from build123d import *

# Parameters (mm, degrees)
F1_DEPTH    = 2.54
F2_R        = 1.905
F3_T2_ANGLE = 165.8998366825


# Not quite as in the source:
# - a fillet or chamfer that OpenCascade refuses, or shapes differently, is made with other operations: its cross-section is extruded or revolved along the edge and cut away or added


with BuildPart() as f1:
    # F0 (on Top) → F1 (new body)
    with BuildSketch(Plane.XY):
        with BuildLine():
            Line((0, -6.35), (0, 0))
            Line((0, 0), (-2.9618976002, 7.0207950124))
            ThreePointArc((-2.9618976002, 7.0207950124), (-5.171443726, -0.4821206784), (0, -6.35))
        make_face()
    extrude(amount=F1_DEPTH)

    # F2
    f2_edges = [f1.edges().sort_by_distance(p)[0] for p in [
        (-5.171444, -0.482121, 2.54),
    ]]
    fillet(f2_edges, radius=F2_R)

    # F3: fillet of radius 1.905 on 1 edges, made by hand

    # F3_s1 → F3_t2 (revolve, cut)
    with BuildSketch(Plane(origin=(2.823536152, 1.0021154347, 0), x_dir=(0, 0, 1), z_dir=(0.942405074, 0.3344737307, 0))):
        with BuildLine():
            ThreePointArc((0.635, -8.3742865468), (0.1659808799, -7.7320963745), (0, -6.9543833811))
            Line((0, -6.9543833811), (0, -8.3742865468))
            Line((0, -8.3742865468), (0.635, -8.3742865468))
        make_face()
    revolve(axis=Axis((2.7291622611, 1.2680210216, 0), (0, 0, 1)), revolution_arc=F3_T2_ANGLE, mode=Mode.SUBTRACT)


solid = f1.part
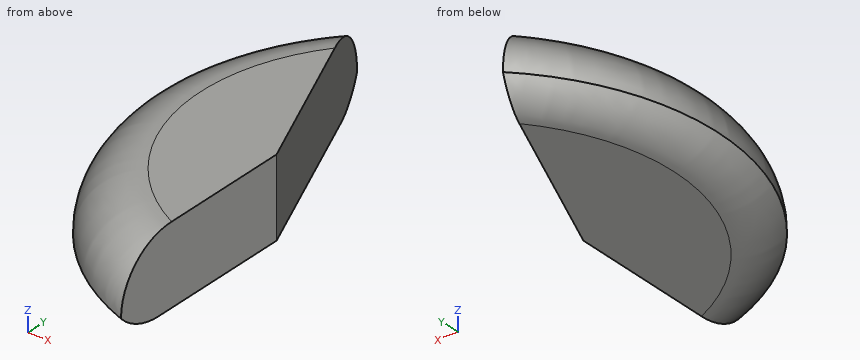
Model file for the job. Use its own axes, mm. Give positions to 0.01 mm unless a question says otherwise; leave off trailing zeros. Loops run counter-clockwise (first coordinate to the right, second up) from the corner with the lowest first, then second, coordinate; pieces in that order, holes last. Notation, with made-up numbers: (44.25, -15.75) - (65.25, -15.75) arc R27 cw to (65.25, 3.25) - close; hole circle Ø6 at (7, 20). An arc over 180 degrees is marked (long way). Use one line per item in the form item = value.
(1) Drill centre lines: L1, parallel to Y at x = -2.8, z = 1.9; L2, parallel to Y at x = -2.6, z = 0.9; L3, parallel to X at y = -2.5, z = 1.3. Where is each one in solid material? Low to high.
Determined:
L1 = -3.96 to 6.5
L2 = -4.8 to 6.16
L3 = -4.3 to 0
(2) Cut at B-B (z = 0.2). Give the cut face in (x, y), then the cut area to 3 significant figures.
Determined:
outline = (-2.72, 6.45) arc R7.52 ccw to (0, -5.74) - (0, 0) - close
area = 37.1 mm^2
(3) Cut at A-A (z = 2.3). Give the cut face in (x, y), then the cut area to 3 significant figures.
Determined:
outline = (-2.55, 6.04) arc R7.11 ccw to (0, -5.3) - (0, 0) - close
area = 31.3 mm^2
(4) Drop a flat-ended pin along its axis: P1, Ø1.5, axis at y = 2.5, z = 1, coming from the +X side. Give the stop position or say it passes through.
Determined:
P1 = -0.74
